from build123d import *

# Parameters (mm, degrees)
F0_R     = 6.35
F0_R_2   = 12.7
F1_DEPTH = 25.4


with BuildPart() as f1:
    # F0 (on Front) → F1 (new body)
    with BuildSketch(Plane.XZ):
        with BuildLine():
            ThreePointArc((-12.984713, 51.275665), (-25.311381, 25.502333), (-51.084713, 13.175665))
            ThreePointArc((-51.084713, 13.175665), (-63.784713, 0.475665), (-51.084713, -12.224335))
            ThreePointArc((-51.084713, -12.224335), (-25.266476, -24.506099), (-12.984713, -50.324335))
            ThreePointArc((-12.984713, -50.324335), (-0.284713, -63.024335), (12.415287, -50.324335))
            ThreePointArc((12.415287, -50.324335), (24.697063, -24.506111), (50.515287, -12.224335))
            ThreePointArc((50.515287, -12.224335), (63.215287, 0.475665), (50.515287, 13.175665))
            ThreePointArc((50.515287, 13.175665), (24.697074, 25.457452), (12.415287, 51.275665))
            ThreePointArc((12.415287, 51.275665), (-0.284713, 63.975665), (-12.984713, 51.275665))
        make_face()
        with Locations((-0.284713, -50.324335)):
            Circle(F0_R, mode=Mode.SUBTRACT)
        with Locations((-51.084713, 0.475665)):
            Circle(F0_R, mode=Mode.SUBTRACT)
        with Locations((-0.284713, 0.475665)):
            Circle(F0_R_2, mode=Mode.SUBTRACT)
        with Locations((-0.284713, 51.275665)):
            Circle(F0_R, mode=Mode.SUBTRACT)
        with Locations((50.515287, 0.475665)):
            Circle(F0_R, mode=Mode.SUBTRACT)
    extrude(amount=F1_DEPTH)


solid = f1.part
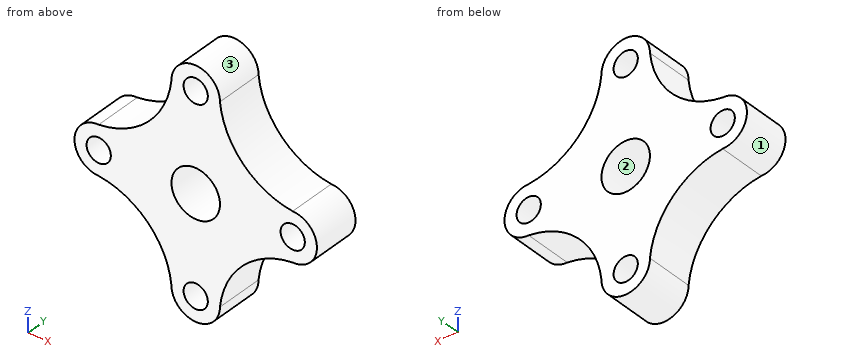
Verification items for the finished model (mm, model axes). Face numbers are marked on the shaded views. Coordinates: 2 decimals unless noted, no trailing zeros. Write each loop counter-clockwise with the first axis right and the second up, starting at its lowest first coordinate (ties: lowest second). Pieces come first, ordered by that corner, then holes. Notation, with made-up numbers: (-10.75, 64) - (33.25, 64) arc R25 ccw to (33.25, 95) - close; hole circle Ø4 at (78, 63). An arc over 180 degrees is marked (long way). Answer as a JSON object with one key per item and string values.
(1) Cross-section at C-C on z = 32.5. Record the cut outline in (x, y).
Report:
{"outline": "(-19.65, -25.4) - (19.01, -25.4) - (19.01, 0) - (-19.65, 0) - close"}
(2) Mould release check, pull along X, two halves, no side actions. Record for the marked faces 1, 2 and 3: pulls with the +X half, pulls with the -X half, needs draft (parallel to the pull), parting line crosses it, or undercut.
Report:
{"face 1": "pulls with the -X half", "face 2": "undercut", "face 3": "parting line crosses it"}
(3) Cross-section at A-A on y = -20. Record the cut outline in (x, z).
Report:
{"outline": "(-51.08, -12.22) arc R42.7 cw to (-12.98, -50.32) arc R12.7 ccw to (12.42, -50.32) arc R42.7 cw to (50.52, -12.22) arc R12.7 ccw to (50.52, 13.18) arc R42.7 cw to (12.42, 51.28) arc R12.7 ccw to (-12.98, 51.28) arc R42.92 cw to (-51.08, 13.18) arc R12.7 ccw to start; hole circle Ø12.7 at (-51.08, 0.48); hole circle Ø25.4 at (-0.28, 0.48); hole circle Ø12.7 at (-0.28, -50.32); hole circle Ø12.7 at (-0.28, 51.28); hole circle Ø12.7 at (50.52, 0.48)"}
(4) Cross-section at B-B on x = -2. Record the cut outline in (y, z), plus the area to 3 significant figures.
Report:
{"outline": "(-25.4, -62.91) - (0, -62.91) - (0, -56.44) - (-25.4, -56.44) - close; (-25.4, -44.21) - (0, -44.21) - (0, -12.11) - (-25.4, -12.11) - close; (-25.4, 13.06) - (0, 13.06) - (0, 45.16) - (-25.4, 45.16) - close; (-25.4, 57.39) - (0, 57.39) - (0, 63.86) - (-25.4, 63.86) - close", "area": "1,960 mm^2"}
(5) Cross-section at D-D on x = -39.5. Record the cut outline in (y, z), plus the area to 3 significant figures.
Report:
{"outline": "(-25.4, -15.09) - (0, -15.09) - (0, 16.09) - (-25.4, 16.09) - close", "area": "792 mm^2"}
(6) Thickness scan on line 1 along Z through (x, y) = (0, -9.25); line 2 along X through (y, z) = (-24, 1); line 3 along Z through (x, y) = (-51, -13.5). Record the ranges inside material, lowest first.
Report:
{"line 1": "-63.02 to -56.67, -43.98 to -12.22, 13.17 to 44.93, 57.62 to 63.97", "line 2": "-63.77 to -57.41, -44.76 to -12.97, 12.4 to 44.19, 56.84 to 63.2", "line 3": "-12.23 to -5.87, 6.83 to 13.18"}
(7) Gauge pin test, flat ends, axial feed: pin 1 Ø3 at (y, z) = (-19.5, -48) entering from +X; pin 2 Ø4 at (x, y) = (44, -21.5) entering from -Z; pin 3 Ø3 at (x, y) = (7, -17.5) entering from -Z. Record the tip position at first contact, or that the pin passes through.
Report:
{"pin 1": "x = 12.99", "pin 2": "z = -13.99", "pin 3": "z = -61.63"}
